Autodesk Inventor part; units mm, degrees
ref_plane "YZ Plane" through (0, 0, 0) normal (1, 0, 0) x (0, 1, 0)
ref_plane "XZ Plane" through (0, 0, 0) normal (0, 1, 0) x (-1, 0, 0)
ref_plane "XY Plane" through (0, 0, 0) normal (0, 0, 1) x (1, 0, 0)
sketch "스케치2" plane through (0, 0, 0) normal (0, 0, 1) x (1, 0, 0)
  line L0 (-42.5, 28) -> (42.5, 28)
  line L1 (42.5, 28) -> (42.5, -28)
  line L2 (42.5, -28) -> (-42.5, -28)
  line L3 (-42.5, -28) -> (-42.5, 28)
  line L4 (-42.5, 28) -> (42.5, -28) construction
  line L5 (42.5, 28) -> (-42.5, -28) construction
  point P0 (0, 0)
  dimension "d6" = 85
  dimension "d7" = 56
extrude "돌출2" add sketch "스케치2" along normal blind 7.65
sketch "스케치4" plane through (0, 0, 0) normal (0, 0, -1) x (-1, 0, 0)
  line L0 (30, 27.091) -> (35, 27.091)
  line L1 (35, 27.091) -> (35, 22.091)
  line L2 (35, 22.091) -> (30, 22.091)
  line L3 (30, 22.091) -> (30, 27.091)
  line L4 (30, 27.091) -> (35, 22.091) construction
  line L5 (35, 27.091) -> (30, 22.091) construction
  line L6 (-42.5, 28) -> (42.5, 28)
  line L7 (-42.5, -28) -> (-42.5, 28)
  line L8 (30.95, 25.541) -> (31.55, 25.541)
  line L9 (31.55, 25.541) -> (31.55, 26.141)
  line L10 (31.55, 26.141) -> (30.95, 26.141)
  line L11 (30.95, 26.141) -> (30.95, 25.541)
  line L12 (30.95, 25.541) -> (31.55, 26.141) construction
  line L13 (31.55, 25.541) -> (30.95, 26.141) construction
  line L14 (32.5, 24.591) -> (32.5, 25.0687)
  line L15 (32.5, 24.591) -> (32.0223, 24.591)
  line L16 (34.05, 25.541) -> (33.45, 25.541)
  line L17 (33.45, 25.541) -> (33.45, 26.141)
  line L18 (33.45, 26.141) -> (34.05, 26.141)
  line L19 (34.05, 26.141) -> (34.05, 25.541)
  line L20 (34.05, 25.541) -> (33.45, 26.141) construction
  line L21 (33.45, 25.541) -> (34.05, 26.141) construction
  line L22 (30.95, 23.641) -> (31.55, 23.641)
  line L23 (31.55, 23.641) -> (31.55, 23.041)
  line L24 (31.55, 23.041) -> (30.95, 23.041)
  line L25 (30.95, 23.041) -> (30.95, 23.641)
  line L26 (30.95, 23.641) -> (31.55, 23.041) construction
  line L27 (31.55, 23.641) -> (30.95, 23.041) construction
  line L28 (34.05, 23.641) -> (33.45, 23.641)
  line L29 (33.45, 23.641) -> (33.45, 23.041)
  line L30 (33.45, 23.041) -> (34.05, 23.041)
  line L31 (34.05, 23.041) -> (34.05, 23.641)
  line L32 (34.05, 23.641) -> (33.45, 23.041) construction
  line L33 (33.45, 23.641) -> (34.05, 23.041) construction
  line L34 (42.5, 28) -> (42.5, -28)
  line L35 (12.5, 22.091) -> (2.5, 22.091)
  line L36 (2.5, 22.091) -> (2.5, 27.091)
  line L37 (2.5, 27.091) -> (12.5, 27.091)
  line L38 (12.5, 27.091) -> (12.5, 22.091)
  line L39 (12.5, 22.091) -> (2.5, 27.091) construction
  line L40 (2.5, 22.091) -> (12.5, 27.091) construction
  line L41 (11.55, 23.641) -> (10.95, 23.641)
  line L42 (10.95, 23.641) -> (10.95, 23.041)
  line L43 (10.95, 23.041) -> (11.55, 23.041)
  line L44 (11.55, 23.041) -> (11.55, 23.641)
  line L45 (11.55, 23.641) -> (10.95, 23.041) construction
  line L46 (10.95, 23.641) -> (11.55, 23.041) construction
  line L47 (11.55, 25.541) -> (11.55, 26.141)
  line L48 (10.95, 26.141) -> (10.95, 25.541)
  line L49 (10.95, 25.541) -> (11.55, 25.541)
  line L50 (11.55, 26.141) -> (10.95, 26.141)
  line L51 (11.55, 26.141) -> (10.95, 25.541) construction
  line L52 (10.95, 26.141) -> (11.55, 25.541) construction
  line L53 (9.05, 23.041) -> (9.05, 23.641)
  line L54 (8.45, 23.641) -> (8.45, 23.041)
  line L55 (8.45, 23.041) -> (9.05, 23.041)
  line L56 (9.05, 23.641) -> (8.45, 23.641)
  line L57 (9.05, 23.641) -> (8.45, 23.041) construction
  line L58 (8.45, 23.641) -> (9.05, 23.041) construction
  line L59 (9.05, 25.541) -> (9.05, 26.141)
  line L60 (8.45, 26.141) -> (8.45, 25.541)
  line L61 (8.45, 25.541) -> (9.05, 25.541)
  line L62 (9.05, 26.141) -> (8.45, 26.141)
  line L63 (9.05, 26.141) -> (8.45, 25.541) construction
  line L64 (8.45, 26.141) -> (9.05, 25.541) construction
  line L65 (6.55, 23.041) -> (6.55, 23.641)
  line L66 (5.95, 23.641) -> (5.95, 23.041)
  line L67 (5.95, 23.041) -> (6.55, 23.041)
  line L68 (6.55, 23.641) -> (5.95, 23.641)
  line L69 (6.55, 23.641) -> (5.95, 23.041) construction
  line L70 (5.95, 23.641) -> (6.55, 23.041) construction
  line L71 (6.55, 25.541) -> (6.55, 26.141)
  line L72 (5.95, 26.141) -> (5.95, 25.541)
  line L73 (5.95, 25.541) -> (6.55, 25.541)
  line L74 (6.55, 26.141) -> (5.95, 26.141)
  line L75 (6.55, 26.141) -> (5.95, 25.541) construction
  line L76 (5.95, 26.141) -> (6.55, 25.541) construction
  line L77 (4.05, 23.041) -> (4.05, 23.641)
  line L78 (3.45, 23.641) -> (3.45, 23.041)
  line L79 (3.45, 23.041) -> (4.05, 23.041)
  line L80 (4.05, 23.641) -> (3.45, 23.641)
  line L81 (4.05, 23.641) -> (3.45, 23.041) construction
  line L82 (3.45, 23.641) -> (4.05, 23.041) construction
  line L83 (4.05, 25.541) -> (4.05, 26.141)
  line L84 (3.45, 26.141) -> (3.45, 25.541)
  line L85 (3.45, 25.541) -> (4.05, 25.541)
  line L86 (4.05, 26.141) -> (3.45, 26.141)
  line L87 (4.05, 26.141) -> (3.45, 25.541) construction
  line L88 (3.45, 26.141) -> (4.05, 25.541) construction
  point P0 (0, 0)
  point P1 (31.25, 25.841)
  point P2 (33.75, 25.841)
  point P3 (31.25, 23.341)
  point P4 (33.75, 23.341)
  point P5 (7.5, 24.591)
  point P6 (11.25, 23.341)
  point P7 (11.25, 25.841)
  point P8 (8.75, 23.341)
  point P9 (8.75, 25.841)
  point P10 (6.25, 23.341)
  point P11 (6.25, 25.841)
  point P12 (3.75, 23.341)
  point P13 (3.75, 25.841)
  dimension "d12" = 5
  dimension "d13" = 5
  dimension "d14" = 0.6
  dimension "d15" = 0.6
  dimension "d18" = 1.25
  dimension "d19" = 7.5
  dimension "d20" = 0.909
  dimension "d21" = 5
  dimension "d22" = 10
  dimension "d23" = 17.5
  dimension "d24" = 0.909
  dimension "d25" = 0.6
  dimension "d26" = 0.6
  dimension "d27" = 1.25
  dimension "d28" = 1.25
  dimension "d31" = 2.5
  dimension "d34" = 2.5
extrude "돌출3" add sketch "스케치4" along normal blind 13.8
sketch "스케치5" plane through (-42.5, -28, 0) normal (0, -1, 0) x (1, 0, 0)
  line L0 (85, 0) -> (0, 0)
  line L1 (24, 0) -> (39.15, 0)
  line L2 (39.15, 0) -> (39.15, -6.2)
  line L3 (39.15, -6.2) -> (24, -6.2)
  line L4 (24, -6.2) -> (24, 0)
  line L5 (0, 0) -> (0, 7.65)
  line L6 (24, -2.9) -> (24.5, -2.9)
  line L7 (26.5, -0.9) -> (26.5, -0.9)
  line L8 (27, -0.4) -> (36.05, -0.4)
  line L9 (36.55, 0) -> (36.55, -13.8) construction
  line L10 (36.55, -0.9) -> (36.55, -0.9)
  line L11 (38.55, -2.9) -> (39.05, -2.9)
  line L12 (39.05, 0) -> (39.05, -13.8)
  arc A0 (24.5, -2.9) -> (26.5, -0.9) centre (24.5, -0.9) ccw
  arc A1 (36.55, -0.9) -> (38.55, -2.9) centre (38.55, -0.9) ccw
  arc A2 (27, -0.4) -> (26.5, -0.9) centre (27, -0.9) ccw
  arc A3 (36.55, -0.9) -> (36.05, -0.4) centre (36.05, -0.9) ccw
  line L13 (24.5, -2.9) -> (24.5, 0.0781)
  line L14 (38.55, -2.9) -> (38.55, 0)
  point P0 (42.5, 0)
  point P1 (26.5, -2.9)
  point P2 (26.5, -0.4)
  point P3 (36.55, -2.9)
  point P4 (36.55, -0.9)
  point P5 (26.5, -0.9)
  point P6 (24.5, 0)
  point P7 (39.05, -6.2)
  dimension "d37" = 24
  dimension "d38" = 15.15
  dimension "d39" = 6.2
  dimension "d40" = 2.5
  dimension "d41" = 2.5
  dimension "d42" = 3.3
  dimension "d43" = 2.5
  dimension "d44" = 2
  dimension "d45" = 0.5
extrude "돌출4" add sketch "스케치5" against normal blind 12.1 contours L12 L11 L14 L0 | L12 L3 L4 L6 A0 A2 L8 A3 A1 L11 | L13 L6 L4 L0
fillet "모깎기1" radius 1 2 edges at (-18.5, -21.95, -6.2) (-3.45, -21.95, -6.2)
extrude "돌출5" cut sketch "스케치5" against normal blind 1 contours L12 L11 L14 L0 | L13 L6 L4 L0
sketch "스케치6" plane through (-15.5, -28, -0.4) normal (0, -1, 0) x (1, 0, 0)
  line L0 (12.05, -2.5) -> (11.55, -2.5)
  arc A0 (9.55, -0.5) -> (11.55, -2.5) centre (11.55, -0.5) ccw
  arc A1 (9.55, -0.5) -> (9.05, 0) centre (9.05, -0.5) ccw
  line L1 (9.05, 0) -> (0, 0)
  arc A2 (0, 0) -> (-0.5, -0.5) centre (0, -0.5) ccw
  arc A3 (-2.5, -2.5) -> (-0.5, -0.5) centre (-2.5, -0.5) ccw
  line L2 (-2.5, -2.5) -> (-3, -2.5)
  line L3 (-3, -2.5) -> (-3, -4.8)
  arc A4 (-3, -4.8) -> (-2, -5.8) centre (-2, -4.8) ccw
  line L4 (-2, -5.8) -> (11.05, -5.8)
  arc A5 (11.05, -5.8) -> (12.05, -4.8) centre (11.05, -4.8) ccw
  line L5 (12.05, -4.8) -> (12.05, -2.5)
  line L6 (-2.5, -4.8) -> (-2.5, -3)
  line L7 (-2.5, -3) -> (-2.5, -3)
  arc A6 (-2.5, -3) -> (0, -0.5) centre (-2.5, -0.5) ccw
  line L8 (0, -0.5) -> (9.05, -0.5)
  arc A7 (9.05, -0.5) -> (11.55, -3) centre (11.55, -0.5) ccw
  line L9 (11.55, -3) -> (11.55, -3)
  line L10 (11.55, -3) -> (11.55, -4.8)
  arc A8 (11.05, -5.3) -> (11.55, -4.8) centre (11.05, -4.8) ccw
  line L11 (11.05, -5.3) -> (-2, -5.3)
  arc A9 (-2.5, -4.8) -> (-2, -5.3) centre (-2, -4.8) ccw
  point P0 (15.5, 0.4)
  point P1 (11.55, -3)
  point P2 (9.05, -0.5)
  point P3 (0, -0.5)
  point P4 (-2.5, -3)
  dimension "d51" = 0.5
extrude "돌출6" cut sketch "스케치6" against normal blind 11.5 contours L6 A6 L8 A7 L10 A8 L11 A9
sketch "스케치7" plane through (-15.5, -28, -0.4) normal (0, -1, 0) x (1, 0, 0)
  arc A0 (9.05, -0.5) -> (11.55, -3) centre (11.55, -0.5) ccw
  line L0 (11.55, -3) -> (11.55, -4.8)
  arc A1 (11.05, -5.3) -> (11.55, -4.8) centre (11.05, -4.8) ccw
  line L1 (11.05, -5.3) -> (-2, -5.3)
  arc A2 (-2.5, -4.8) -> (-2, -5.3) centre (-2, -4.8) ccw
  line L2 (-2.5, -4.8) -> (-2.5, -3)
  arc A3 (-2.5, -3) -> (0, -0.5) centre (-2.5, -0.5) ccw
  line L3 (0, -0.5) -> (9.05, -0.5)
  line L4 (12.05, -2.5) -> (11.55, -2.5)
  arc A4 (9.55, -0.5) -> (11.55, -2.5) centre (11.55, -0.5) ccw
  arc A5 (9.55, -0.5) -> (9.05, 0) centre (9.05, -0.5) ccw
  line L5 (9.05, 0) -> (0, 0)
  arc A6 (0, 0) -> (-0.5, -0.5) centre (0, -0.5) ccw
  arc A7 (-2.5, -2.5) -> (-0.5, -0.5) centre (-2.5, -0.5) ccw
  line L6 (-2.5, -2.5) -> (-3, -2.5)
  line L7 (-3, -2.5) -> (-3, -4.8)
  arc A8 (-3, -4.8) -> (-2, -5.8) centre (-2, -4.8) ccw
  line L8 (-2, -5.8) -> (11.05, -5.8)
  arc A9 (11.05, -5.8) -> (12.05, -4.8) centre (11.05, -4.8) ccw
  line L9 (12.05, -4.8) -> (12.05, -2.5)
  point P0 (15.5, 0.4)
extrude "돌출7" add sketch "스케치7" along normal blind 0.7
sketch "스케치9" plane through (0, 0, 7.65) normal (0, 0, 1) x (1, 0, 0)
  line L0 (-42.5753, 28.643) -> (43.0741, 28.643) construction
  line L1 (43.0741, 28.643) -> (43.0741, -28.4566) construction
  line L2 (43.0741, -28.4566) -> (-42.5753, -28.4566) construction
  line L3 (-42.5753, -28.4566) -> (-42.5753, 28.643) construction
properties part number "lcd 디스플레이"
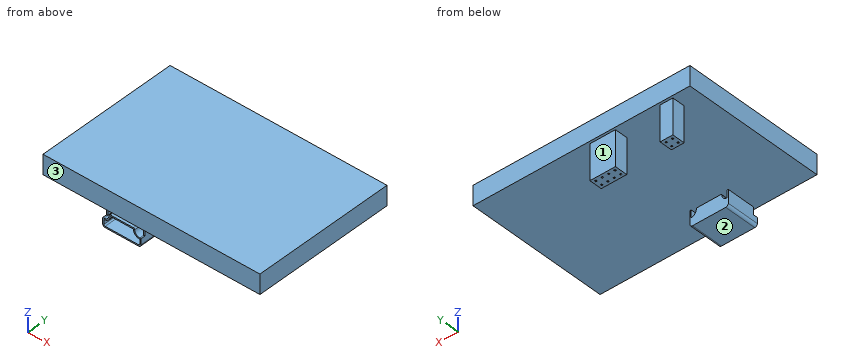
Design review of the part built by this model. Coordinates are the model's own, in mm. Face numbers are marked on the shaded views. A direction names the side the tool comes from. Give positions to 0.01 mm unless a question says otherwise; leave off trailing zeros. Order: outer loops, then holes, each group sorted by start corner. A loop starts at its lowest first (then second) coordinate and runs counter-clockwise, first axis right, second up.
1. Add section A-A, the plane y = -21.5. State the section outline as (x, z) points.
Solution:
outline: (-42.5, 0) - (-18.5, 0) - (-18.5, -5.2) arc R1 ccw to (-17.5, -6.2) - (-4.45, -6.2) arc R1 ccw to (-3.45, -5.2) - (-3.45, 0) - (42.5, 0) - (42.5, 7.65) - (-42.5, 7.65) - close; hole (-18, -5.2) arc R0.5 ccw to (-17.5, -5.7) - (-4.45, -5.7) arc R0.5 ccw to (-3.95, -5.2) - (-3.95, -3.4) arc R2.5 cw to (-6.45, -0.9) - (-15.5, -0.9) arc R2.5 cw to (-18, -3.4) - close; hole (-18, -2.9) arc R2 ccw to (-16, -0.9) arc R0.5 cw to (-15.5, -0.4) - (-6.45, -0.4) arc R0.5 cw to (-5.95, -0.9) arc R2 ccw to (-3.95, -2.9) - (-3.95, 0) - (-18, 0) - close
2. Add section D-D, the plane y = 18. State the section outline as (x, z) points, then the cut area to 3 significant figures.
Solution:
outline: (-42.5, 0) - (42.5, 0) - (42.5, 7.65) - (-42.5, 7.65) - close
area: 650 mm2
3. Add section B-B, the plane z = -9. State how many separate pieces and enclosed holes the cut face has, then the cut area to 3 significant figures.
Solution:
separate pieces: 2
enclosed holes: 12
area: 70.7 mm2
4. To check wall thickness, follow L1, parallel to Y at x = -31, z = -12.5; L2, parallel to Y at x = -9.5, z = -3; L3, parallel to X at y = -24.5, z = -1.5. State the ranges of each line that lie inside material, in increasing order.
Solution:
L1: y = 22.09 to 23.04, 23.64 to 25.54, 26.14 to 27.09
L2: y = -16.5 to -15.9, 22.09 to 27.09
L3: x = -18.5 to -18, -16.09 to -15.57, -6.38 to -5.86, -3.95 to -3.45
5. For pin 1 Ø4 at (x, z) = (-31.5, -9) entering from +Y; pin 2 Ø6 at (x, y) = (15.5, 6) entering from -Z; pin 3 Ø0.5 at (y, z) = (26, -6) entering from +X, all flat-tipped, find the tip position at first contact; note any pin that passes through.
Solution:
pin 1: stops at y = 27.09
pin 2: stops at z = 0
pin 3: stops at x = -2.5
6. Add section C-C, the plane x = 21.5. State the section outline as (y, z) points.
Solution:
outline: (-28, 0) - (28, 0) - (28, 7.65) - (-28, 7.65) - close
7. Tool access review of the marked faces 1, 2 and 3: name each direction out of +Z, -Z, +X, -X, +Y, -Y from which nothing blocks a thin tool from reaching the whole face with its end or side.
Solution:
face 1: -Z, +X, -X, +Y
face 2: -Z, +X, -X, -Y
face 3: +Z, +X, -X, -Y
